Read the model definition and answer for the solid it produces. Units are mm, in the model's axes. A direction names the side the tool comes from. Coordinates: 2 decimals unless noted, no trailing zeros. Loops run counter-clockwise (first coordinate to the right, second up) from the corner with the lowest first, then second, coordinate; pieces in that order, holes last. Notation, with made-up numbers: (2, 64) -> (22, 64) arc R23 cw to (22, 89) -> close; hole circle Ø4 at (74.5, 82). An arc over 180 degrees is marked (long way). Answer in a Markdown table with one row per item.
```python
from build123d import *

# Parameters (mm, degrees)
SKETCH1_W           = 23.622
SKETCH1_H           = 12.192
BOSS_EXTRUDE1_DEPTH = 20.32
SKETCH2_R           = 5.080697271
BOSS_EXTRUDE2_DEPTH = 2.032
SKETCH3_W           = 12.192
SKETCH3_H           = 1.5875
BOSS_EXTRUDE3_DEPTH = 4.7625
CUT_EXTRUDE1_REACH  = 26.613
SKETCH5_R           = 1.0795
FILLET1_R           = 0.508


with BuildPart() as part:
    # Sketch1 → Boss-Extrude1 (new body)
    with BuildSketch(Plane(origin=(0, 0, 0), x_dir=(1, 0, 0), z_dir=(0, 1, 0))):
        Rectangle(SKETCH1_W, SKETCH1_H)
    extrude(amount=BOSS_EXTRUDE1_DEPTH)

    # Sketch2 → Boss-Extrude2 (add)
    with BuildSketch(Plane(origin=(0, 20.32, 0), x_dir=(1, 0, 0), z_dir=(0, 1, 0))):
        with Locations((5.378708036, 0)):
            Circle(SKETCH2_R)
        with BuildLine():
            ThreePointArc((0.966939793, -2.519878116), (0.298010766, 0), (0.966939793, 2.519878116))
            ThreePointArc((0.966939793, 2.519878116), (-2.454485361, 0), (0.966939793, -2.519878116))
        make_face()
    extrude(amount=BOSS_EXTRUDE2_DEPTH)

    # Sketch3 → Boss-Extrude3 (add)
    with BuildSketch(Plane(origin=(11.811, 0, 0), x_dir=(0, 0, -1), z_dir=(1, 0, 0))):
        with Locations((0, 16.35125)):
            Rectangle(SKETCH3_W, SKETCH3_H)
    boss_extrude3 = extrude(amount=BOSS_EXTRUDE3_DEPTH)

    # Sketch5 → Cut-Extrude1 (cut, up to next)
    with BuildSketch(Plane(origin=(0, 17.145, 0), x_dir=(1, 0, 0), z_dir=(0, 1, 0)), mode=Mode.PRIVATE) as cut_extrude1_sk1:
        with Locations(Location((14.19225, 0, 0), (0, 0, 270))):
            Circle(SKETCH5_R)
    cut_extrude1_tool1 = extrude(cut_extrude1_sk1.sketch, amount=-CUT_EXTRUDE1_REACH, mode=Mode.PRIVATE) & part.part
    cut_extrude1 = cut_extrude1_tool1.solids().sort_by_distance((14.19225, 17.145, 0))[0]
    add(cut_extrude1, mode=Mode.SUBTRACT)

    # Mirror1: Boss-Extrude3, Cut-Extrude1 across plane
    add(boss_extrude3.mirror(Plane(origin=(0, 0, 0), x_dir=(0, 0, 1), z_dir=(1, 0, 0))))
    add(cut_extrude1.mirror(Plane(origin=(0, 0, 0), x_dir=(0, 0, 1), z_dir=(1, 0, 0))), mode=Mode.SUBTRACT)

    # Fillet1
    fillet1_edges = [part.edges().sort_by_distance(p)[0] for p in [
        (16.5735, 16.35125, 6.096),
        (16.5735, 16.35125, -6.096),
        (-16.5735, 16.35125, 6.096),
        (-16.5735, 16.35125, -6.096),
    ]]
    fillet(fillet1_edges, radius=FILLET1_R)


solid = part.part
```
1. Find the intervals of material crossed by probe 1 along X at (y, z) = (16.15, 0); probe 2 along X at (y, z) = (19, 3.75); probe 3 along Y at (x, z) = (13.5, 3.5) (1 decimal), in increasing order.
A:
| item | result |
|---|---|
| probe 1 | x = -16.57 to -15.27, -13.11 to 13.11, 15.27 to 16.57 |
| probe 2 | x = -11.81 to 11.81 |
| probe 3 | y = 15.6 to 17.1 |
2. A cutting plane is placed at C-C on z = -1.5. Give the vertices of the cut face in (x, y) (1 decimal).
A:
| item | result |
|---|---|
| outline | (-16.6, 15.6) -> (-11.8, 15.6) -> (-11.8, 0) -> (11.8, 0) -> (11.8, 15.6) -> (16.6, 15.6) -> (16.6, 17.1) -> (11.8, 17.1) -> (11.8, 20.3) -> (10.2, 20.3) -> (10.2, 22.4) -> (-2, 22.4) -> (-2, 20.3) -> (-11.8, 20.3) -> (-11.8, 17.1) -> (-16.6, 17.1) -> close |
3. A cutting plane is placed at B-B on x = -13.5. Give the vertices of the cut face in (y, z) (1 decimal), and give its area (3 significant figures).
A:
| item | result |
|---|---|
| outline | (15.6, -6.1) -> (17.1, -6.1) -> (17.1, -0.8) -> (15.6, -0.8) -> close; (15.6, 0.8) -> (17.1, 0.8) -> (17.1, 6.1) -> (15.6, 6.1) -> close |
| area | 16.7 mm2 |
4. A tool of negligible diameter and unlimited length cuts with its end or side. For faces 4 (the flat face through (-11.811, 8, 0)), 5 (the flat face through (-14.2, 17.145, 1.4)), 6 (the flat face through (14.2, 17.145, 1.4)), from which of +Z, -Z, +X, -X, +Y, -Y can it reach the whole face along a straight path? Write none if from no direction.
A:
| item | result |
|---|---|
| face 4 | +Z, -Z, -X, -Y |
| face 5 | +Z, -Z, -X, +Y |
| face 6 | +Z, -Z, +X, +Y |
5. The mould has two halves that part along Z. Classify faces 1 (the cylindrical face through (-15.263, 16.362, -0.141)), 2 (the flat face through (-3, 20.32, 0)), 3 (the cylindrical face through (10.456, 21.322, 0.187)): pulls with the +Z half, pulls with the -Z half, needs draft (parallel to the pull), parting line crosses it, or undercut.
A:
| item | result |
|---|---|
| face 1 | undercut |
| face 2 | needs draft |
| face 3 | parting line crosses it |
6. A cutting plane is placed at A-A on z = 0. Give the vertices of the cut face in (x, y) (1 decimal).
A:
| item | result |
|---|---|
| outline | (-16.6, 15.6) -> (-15.3, 15.6) -> (-15.3, 17.1) -> (-16.6, 17.1) -> close; (-13.1, 15.6) -> (-11.8, 15.6) -> (-11.8, 0) -> (11.8, 0) -> (11.8, 15.6) -> (13.1, 15.6) -> (13.1, 17.1) -> (11.8, 17.1) -> (11.8, 20.3) -> (10.5, 20.3) -> (10.5, 22.4) -> (-2.5, 22.4) -> (-2.5, 20.3) -> (-11.8, 20.3) -> (-11.8, 17.1) -> (-13.1, 17.1) -> close; (15.3, 15.6) -> (16.6, 15.6) -> (16.6, 17.1) -> (15.3, 17.1) -> close |
7. Given pin 1 Ø1 at (y, z) = (18.5, 3) entering from -X; pin 2 Ø2.5 at (x, z) = (14.19, 0) entering from +Y (3 decimals); pin 3 Ø3.5 at (x, z) = (-5, 1.5) entering from +Y, each flat-ended and moving along its own axis, determine where each tip first touches the part or whether it passes through.
A:
| item | result |
|---|---|
| pin 1 | stops at x = -11.81 |
| pin 2 | stops at y = 17.145 |
| pin 3 | stops at y = 20.32 |
8. A cutting plane is placed at D-D on y = 15. Give the vertices of the cut face in (x, z).
A:
| item | result |
|---|---|
| outline | (-11.81, -6.1) -> (11.81, -6.1) -> (11.81, 6.1) -> (-11.81, 6.1) -> close |
